Model file for the job. Use its own axes, mm. A direction names the side the tool comes from. Give positions to 0.01 mm unless a question says otherwise; leave off trailing zeros. Write each loop counter-clockwise with the first axis right and the second up, starting at its lowest first coordinate (ties: lowest second). Pieces come first, ordered by that corner, then holes.
```python
from build123d import *

# Parameters (mm, degrees)
SKETCH1_W           = 40
SKETCH1_H           = 16
BOSS_EXTRUDE1_DEPTH = 13.3
CUT_EXTRUDE2_DEPTH  = 11.5
SKETCH3_R           = 3.5
CUT_EXTRUDE3_DEPTH  = 24.8
SKETCH4_W           = 21
SKETCH4_H           = 12
CUT_EXTRUDE4_DEPTH  = 4
SKETCH5_W           = 100
SKETCH5_H           = 20
BOSS_EXTRUDE2_DEPTH = 2
SKETCH6_W           = 100
SKETCH6_H           = 20
BOSS_EXTRUDE3_DEPTH = 2
SKETCH7_R           = 4
CUT_EXTRUDE5_DEPTH  = 2
CUT_EXTRUDE8_REACH  = 104.004
SKETCH8_R           = 3.5
FILLET1_R           = 0.5
FILLET2_R           = 0.5
SKETCH9_R           = 3.5
BOSS_EXTRUDE4_DEPTH = 3
SKETCH10_R          = 1.5
CUT_EXTRUDE9_DEPTH  = 104.274827523


with BuildPart() as part:
    # Sketch1 → Boss-Extrude1 (new body)
    with BuildSketch(Plane(origin=(0, 0, 0), x_dir=(1, 0, 0), z_dir=(0, 1, 0))):
        Rectangle(SKETCH1_W, SKETCH1_H)
    extrude(amount=BOSS_EXTRUDE1_DEPTH)

    # Sketch2 → Cut-Extrude2 (cut)
    with BuildSketch(Plane.XZ):
        with BuildLine():
            ThreePointArc((-4.245094519, 3.659354296), (-14.835807847, -1.394039732), (-3.104556161, -1.115231786))
            ThreePointArc((-3.104556161, -1.115231786), (-1.705240191, 1.742549665), (-4.245094519, 3.659354296))
        make_face()
    extrude(amount=-CUT_EXTRUDE2_DEPTH, mode=Mode.SUBTRACT)

    # Sketch3 → Cut-Extrude3 (cut)
    with BuildSketch(Plane(origin=(0, 0, 0), x_dir=(-1, 0, 0), z_dir=(0, -1, 0))):
        with Locations(Location((9, 0, 0), (0, 0, 90))):
            Circle(SKETCH3_R)
    extrude(amount=-CUT_EXTRUDE3_DEPTH, mode=Mode.SUBTRACT)

    # Sketch4 → Cut-Extrude4 (cut)
    with BuildSketch(Plane(origin=(0, 0, 0), x_dir=(-1, 0, 0), z_dir=(0, -1, 0))):
        with Locations((4.5, 0)):
            Rectangle(SKETCH4_W, SKETCH4_H)
    extrude(amount=-CUT_EXTRUDE4_DEPTH, mode=Mode.SUBTRACT)

    # Sketch5 → Boss-Extrude2 (add)
    with BuildSketch(Plane(origin=(20, 0, 0), x_dir=(0, 0, -1), z_dir=(1, 0, 0))):
        with Locations((42, 3.3)):
            Rectangle(SKETCH5_W, SKETCH5_H)
    extrude(amount=BOSS_EXTRUDE2_DEPTH)

    # Sketch6 → Boss-Extrude3 (add)
    with BuildSketch(Plane.ZY.offset(20)):
        with Locations((-42, 3.3)):
            Rectangle(SKETCH6_W, SKETCH6_H)
    extrude(amount=BOSS_EXTRUDE3_DEPTH)

    # Sketch7 → Cut-Extrude5 (cut)
    with BuildSketch(Plane(origin=(22, 0, 0), x_dir=(0, 0, -1), z_dir=(1, 0, 0))):
        with Locations((77, 3.206448438)):
            Circle(SKETCH7_R)
    extrude(amount=-CUT_EXTRUDE5_DEPTH, mode=Mode.SUBTRACT)

    # Sketch8 → Cut-Extrude8 (cut, up to next)
    with BuildSketch(Plane(origin=(-20, 0, 0), x_dir=(0, 0, -1), z_dir=(1, 0, 0)), mode=Mode.PRIVATE) as cut_extrude8_sk1:
        with Locations((77, 3.3)):
            Circle(SKETCH8_R)
    cut_extrude8_tool1 = extrude(cut_extrude8_sk1.sketch, amount=-CUT_EXTRUDE8_REACH, mode=Mode.PRIVATE) & part.part
    add(cut_extrude8_tool1.solids().sort_by_distance((-20, 3.3, -77))[0], mode=Mode.SUBTRACT)

    # Fillet1
    fillet1_edges = [part.edges().sort_by_distance(p)[0] for p in [
        (20, 13.3, -50),
        (22, 13.3, -42),
        (-20, 13.3, -50),
        (-22, 13.3, -42),
    ]]
    fillet(fillet1_edges, radius=FILLET1_R)

    # Fillet2
    fillet2_edges = [part.edges().sort_by_distance(p)[0] for p in [
        (21.853553391, 13.153553391, -92),
        (20.146446609, 13.153553391, -92),
        (-20, 3.05, -92),
        (-22, 3.05, -92),
        (-21.853553391, 13.153553391, -92),
        (-20.146446609, 13.153553391, -92),
        (22, 3.05, 8),
        (21.853553391, 13.153553391, 8),
        (-21.853553391, 13.153553391, 8),
        (21, -6.7, 8),
        (20, 3.05, -92),
        (21, -6.7, -92),
        (22, 3.05, -92),
        (-21, -6.7, 8),
        (-21, -6.7, -92),
        (-22, 3.05, 8),
        (0, 13.3, 8),
        (21, 13.3, -92),
        (-21, 13.3, -92),
    ]]
    fillet(fillet2_edges, radius=FILLET2_R)

    # Sketch9 → Boss-Extrude4 (add)
    with BuildSketch(Plane(origin=(0, 13.3, 0), x_dir=(1, 0, 0), z_dir=(0, 1, 0))):
        with Locations(Location((10.5, 0, 0), (0, 0, 270))):
            Circle(SKETCH9_R)
    extrude(amount=BOSS_EXTRUDE4_DEPTH)

    # Sketch10 → Cut-Extrude9 (cut, through all)
    with BuildSketch(Plane.ZY.offset(22)):
        with Locations((-42, 3.05)):
            Circle(SKETCH10_R)
    extrude(amount=-CUT_EXTRUDE9_DEPTH, mode=Mode.SUBTRACT)


solid = part.part
```
1. Pin check, flat tips, straight feed: P1, Ø6.5, axis at x = -11.5, z = -3.5, coming from the -Y side; P2, Ø3, axis at x = -8, y = 1.5, coming from the -Z side; P3, Ø6.5, axis at y = 3.3, z = -77, coming from the -X side; P4, Ø4, axis at y = 3.05, z = -42, coming from the -X side. Stop position of each tip, or through.
Calculated:
P1: stops at y = 0
P2: stops at z = -8
P3: passes through
P4: stops at x = -22
2. Probe probe 1 along X at (y, z) = (9.5, -15); probe 2 along Y at (x, z) = (20.5, -42); probe 3 along Z at (x, y) = (0, 1.25). List the from-to ranges inside material, lowest first.
Calculated:
probe 1: x = -22 to -20, 20 to 22
probe 2: y = -6.7 to 1.55, 4.55 to 13.3
probe 3: z = -8 to -6, 6 to 8
3. Slice it at A-A, the plane y = -3. Write the cut outline in (x, z), and give its area (3 significant figures).
Calculated:
outline: (-22, -91.5) arc R0.5 ccw to (-21.5, -92) - (-20.5, -92) arc R0.5 ccw to (-20, -91.5) - (-20, 8) - (-21.5, 8) arc R0.5 ccw to (-22, 7.5) - close; (20, -91.5) arc R0.5 ccw to (20.5, -92) - (21.5, -92) arc R0.5 ccw to (22, -91.5) - (22, 7.5) arc R0.5 ccw to (21.5, 8) - (20, 8) - close
area: 400 mm2
4. Slice it at D-D, the plane x = -7. Write the cut outline in (y, z).
Calculated:
outline: (0, -8) - (13.3, -8) - (13.3, -2.87) - (11.5, -2.87) - (11.5, -5.66) - (4, -5.66) - (4, -6) - (0, -6) - close; (0, 6) - (4, 6) - (4, 5.66) - (11.5, 5.66) - (11.5, 2.87) - (13.3, 2.87) - (13.3, 7.5) arc R0.5 ccw to (12.8, 8) - (0, 8) - close
5. Which spindle directions (+Z, -Z, +X, -X, +Y, -Y) get a long thin tool onto all of the face, cutting with end or side? Do faces 1 (the flat face through (9, 0, 0)), 2 (the flat face through (-15, 2, 0)), 3 (the cylindrical face through (21.014, 3.382, -73.004)). Say none if no direction does.
Calculated:
face 1: +Z, -Z, -Y
face 2: -Y
face 3: +X
6. Slice it at C-C, the plane z = -19. Write the cut outline in (x, y), and give its area (3 significant figures).
Calculated:
outline: (-22, -6.7) - (-20, -6.7) - (-20, 12.8) arc R0.5 ccw to (-20.5, 13.3) - (-21.5, 13.3) arc R0.5 ccw to (-22, 12.8) - close; (20, -6.7) - (22, -6.7) - (22, 12.8) arc R0.5 ccw to (21.5, 13.3) - (20.5, 13.3) arc R0.5 ccw to (20, 12.8) - close
area: 79.8 mm2
7. Slice it at B-B, the plane z = -77. Write the cut outline in (x, y).
Calculated:
outline: (-22, -6.7) - (-20, -6.7) - (-20, -0.2) - (-22, -0.2) - close; (-22, 6.8) - (-20, 6.8) - (-20, 12.8) arc R0.5 ccw to (-20.5, 13.3) - (-21.5, 13.3) arc R0.5 ccw to (-22, 12.8) - close; (20, -6.7) - (22, -6.7) - (22, -0.79) - (20, -0.79) - close; (20, 7.21) - (22, 7.21) - (22, 12.8) arc R0.5 ccw to (21.5, 13.3) - (20.5, 13.3) arc R0.5 ccw to (20, 12.8) - close
8. Pull direction Z, two halves, no side cores. Call faces 4 (the flat face through (21, -6.7, -41)), 5 (the cylindrical face through (7.083, 14.779, -0.759)), 6 (the flat face through (-4, 2, -6)): +Z half, -Z half, draft (parallel to the pull), parting line (faces both ways), or undercut.
Calculated:
face 4: draft
face 5: parting line
face 6: undercut
